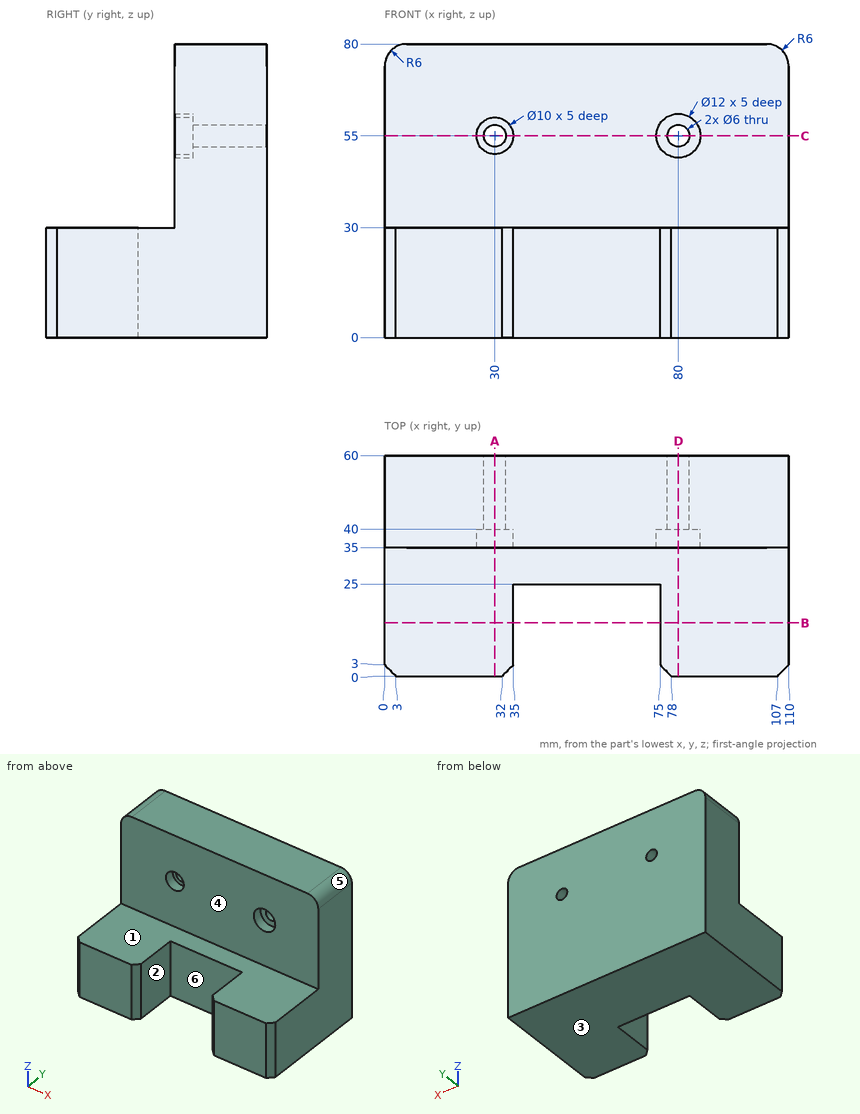
Study the drawing (mm; zero at the part's minimum x, y, z) and answer. A direction names the side the tool comes from. Coordinates: 2 decimals unless noted, no trailing zeros. Write each loop counter-clockwise with the first axis right and the second up, starting at its lowest first coordinate (ties: lowest second). Pieces come first, ordered by that corner, then holes. Notation, with made-up numbers: (28, 6) - (68, 6) arc R34 ccw to (68, 42) - close; hole circle Ø7 at (-15.75, -30). An arc over 180 degrees is marked (long way). Return JSON: item names as keys, results as strings. Group by question number.
1. A cutting plane is placed at A-A, the plane x = 30. Determine the outline of the cut face in (y, z), plus the area to 3 significant figures.
2. A cutting plane is placed at C-C, the plane z = 55. Determine the outline of the cut face in (x, y), plus the area to 3 significant figures.
3. A cutting plane is placed at B-B, the plane y = 14.5. Determine the outline of the cut face in (x, z), plus the area to 3 significant figures.
4. A cutting plane is placed at D-D, the plane x = 80. Determine the outline of the cut face in (y, z).
5. Which of the six approach directions +Z, -Z, +X, -X, +Y, -Y give full straight-line access (tool end or side, diameter ignored) to the marked faces 1, 2 and 3?
6. Straight lines are drawn through the part: L1, parallel to X at y = 54, z = 55; L2, parallel to Z at x = 30, y = 55; L3, parallel to X at y = 3, z = 27. For each, find the intervals that lie inside material, in ascending order.
7. Given pin 1 (25 mm diameter, centred on x = 56, z = 62.5, fed in from -Y); pin 2 (24 mm diameter, centred on x = 57, z = 15.5, fed in from -Y); pin 3 (5 mm diameter, centred on x = 29.5, z = 56, fed in from -Y), each flat-ended and moving along its own axis, determine where each tip first touches the part or whether it passes through.
8. Determine the mould class of the marked faces 4, 5 and 6 for opening direction X: released by +X, released by -X, zero draft, split by the parting line, or undercut.
Ans:
{
 "1": {"outline": "(0, 0) - (60, 0) - (60, 52) - (40, 52) - (40, 50) - (35, 50) - (35, 30) - (0, 30) - close; (35, 60) - (40, 60) - (40, 58) - (60, 58) - (60, 80) - (35, 80) - close", "area": "2,880 mm²"},
 "2": {"outline": "(0, 35) - (25, 35) - (25, 40) - (27, 40) - (27, 60) - (0, 60) - close; (33, 40) - (35, 40) - (35, 35) - (74, 35) - (74, 40) - (77, 40) - (77, 60) - (33, 60) - close; (83, 40) - (86, 40) - (86, 35) - (110, 35) - (110, 60) - (83, 60) - close", "area": "2,400 mm²"},
 "3": {"outline": "(0, 0) - (35, 0) - (35, 30) - (0, 30) - close; (75, 0) - (110, 0) - (110, 30) - (75, 30) - close", "area": "2,100 mm²"},
 "4": {"outline": "(0, 0) - (60, 0) - (60, 52) - (40, 52) - (40, 49) - (35, 49) - (35, 30) - (0, 30) - close; (35, 61) - (40, 61) - (40, 58) - (60, 58) - (60, 80) - (35, 80) - close"},
 "5": {"face 1": "+Z, +X, -X, -Y", "face 2": "+Z, -Z, -Y", "face 3": "-Z, +X, -X, +Y, -Y"},
 "6": {"L1": "0 to 27, 33 to 77, 83 to 110", "L2": "0 to 52, 58 to 80", "L3": "0 to 35, 75 to 110"},
 "7": {"pin 1": "y = 35", "pin 2": "y = 25", "pin 3": "y = 40"},
 "8": {"face 4": "zero draft", "face 5": "released by +X", "face 6": "undercut"}
}
